Can you work these out from the drawing? Everything is in mm from the part's minimum corner. A direction names the side the tool comes from. Give positions to 0.01 mm unless a question says otherwise; leave off trailing zeros. Write each loop counter-clockwise with the first axis right and the second up, starting at its lowest first coordinate (ties: lowest second). Pieces come first, ordered by that corner, then holes. Notation, with made-up numbers: (16.5, 31.25) - (57.5, 31.25) arc R31 cw to (57.5, 64.25) - close; hole circle Ø9 at (37.25, 68). An arc over 180 degrees is marked (long way). Use a Markdown table: item, result. Add a question column.
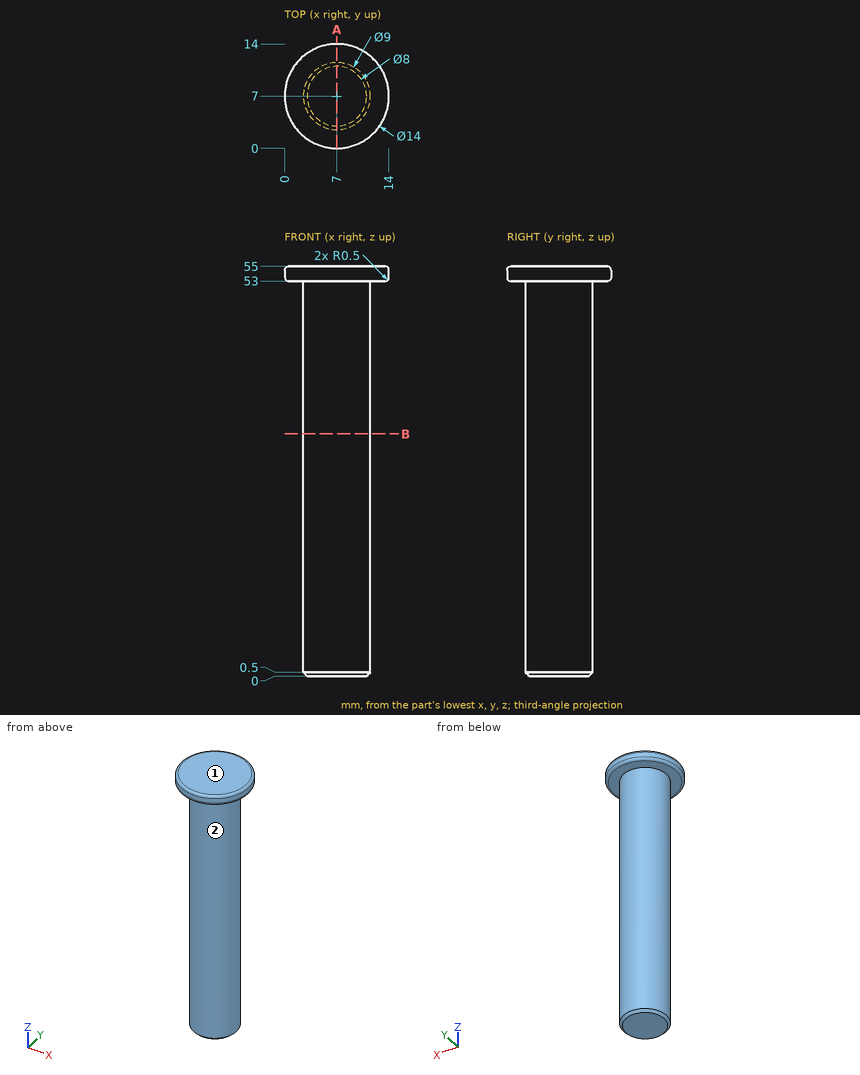
Q1. I'm going to push flat-ended pins straight in: P1, Ø1.5, axis at y = 4.5, z = 16.5, coming from the -X side; P2, Ø4, axis at x = 10, z = 22.5, coming from the +Y side; P3, Ø3, axis at y = 9, z = 20, coming from the -X side; P4, Ø4, axis at x = 7.5, y = 9, coming from the -Z side. Where does each tip first touch, or does it pass through?
Q2. On a 3-axis mill with a long thin cutter (end or side, diameter ignored), from which of +Z, -Z, +X, -X, +Y, -Y can I reach the whole of each face in a straight line? I mean the marked faces 1 and 2. Say none if no direction works.
Q3. Suppose I cut it at A-A (x = 7). Please give me the cut outline in (y, z), and give its area (3 significant figures).
Q4. Suppose I cut it at B-B (z = 32.5). Please give me the cut outline in (x, y), and give its area (3 significant figures).
Q5. If I drill on probe 1 along Z at (x, y) = (5.5, 2.5); probe 2 along Y at (x, z) = (6.75, 9.5), over which ranges is the centre line in solid material (lowest first)? Write a range as [from, to].
Derived:
| question | item | result |
|---|---|---|
| 1 | P1 | x = 2.85 |
| 1 | P2 | y = 11.39 |
| 1 | P3 | x = 2.53 |
| 1 | P4 | z = 0 |
| 2 | face 1 | +Z, +X, -X, +Y, -Y |
| 2 | face 2 | -Z |
| 3 | outline | (0, 53.5) arc R0.5 ccw to (0.5, 53) - (2.5, 53) - (2.5, 0.5) - (3, 0) - (11, 0) - (11.5, 0.5) - (11.5, 53) - (13.5, 53) arc R0.5 ccw to (14, 53.5) - (14, 54.5) arc R0.5 ccw to (13.5, 55) - (0.5, 55) arc R0.5 ccw to (0, 54.5) - close |
| 3 | area | 505 mm² |
| 4 | outline | circle Ø9 at (7, 7) |
| 4 | area | 63.6 mm² |
| 5 | probe 1 | [53, 55] |
| 5 | probe 2 | [2.51, 11.49] |
